Here's how the part is built. I have some questions about the finished solid (model axes, mm). A direction names the side the tool comes from. Round coordinates to 2 decimals unless told otherwise and drop trailing zeros. Loops run counter-clockwise (first coordinate to the right, second up) from the corner with the lowest first, then second, coordinate; pieces in that order, holes last. Notation, with made-up numbers: (6.25, 4.25) - (20.25, 4.25) arc R32 cw to (20.25, 40.25) - close; hole circle Ø2 at (49.5, 77). An arc over 180 degrees is marked (long way). Answer as a JSON object with one key per item and string values. Group by question number.
1) Will these pins go through, and if not, where does the flat tip stop? P1, Ø1.5, axis at y = 1.5, z = 1.5, coming from the -X side; P2, Ø0.9, axis at y = 2, z = 1.5, coming from the +X side; P3, Ø0.8, axis at x = 1.5, z = 1, coming from the -Y side.
2) I want a section at C-C, the plane y = 2.5. Please give me the cut outline in (x, z).
3) Which directions (+Z, -Z, +X, -X, +Y, -Y) give clear straight access to the entire face, cutting with the end or side of a thin tool? Please do faces 1 (the face through (1, 3, 1)), 2 (the face through (0, 14, 1)), 3 (the face through (7.75, 2, 1)).
4) If I drill on line 1 along X through (y, z) = (25, 0.7); line 2 along Y through (x, z) = (6.25, 2.3); line 3 along Y through (x, z) = (4.75, 2.05), over which ranges is the centre line in solid material (lowest first)? Write a range as [from, to].
5) I want a section at D-D, the plane x = 9.75. Please give me the cut outline in (y, z).
6) I want a section at A-A, the plane z = 1.6. Please give me the cut outline in (x, y), then the cut area to 3 significant figures.
7) If we mould it in two halves opening along X, with no side actions, what happens to faces 4 (the face through (9, 3, 1)), 5 (the face through (10.5, 14, 1)), 6 (the face through (5.3, 26.5, 1.5))? For each: pulls with the +X half, pulls with the -X half, needs draft (parallel to the pull), parting line crosses it, or undercut.
8) I want a section at B-B, the plane x = 4.75. Please give me the cut outline in (y, z), then the cut area to 3 significant figures.
from build123d import *

# Parameters (mm, degrees)
PLATE_THICKNESS_3MM_DEPTH = 3


with BuildPart() as part:
    # Sketch1 → Plate_thickness_3mm (new body)
    with BuildSketch(Plane.XY):
        with BuildLine():
            Line((10.5, 25), (10.5, 3))
            Line((10.5, 3), (7.75, 3))
            Line((7.75, 3), (7.75, 0))
            Line((7.75, 0), (2.75, 0))
            Line((2.75, 0), (2.75, 3))
            Line((2.75, 3), (0, 3))
            Line((0, 3), (0, 25))
            ThreePointArc((0, 25), (1.537689399, 28.712310601), (5.25, 30.25))
            ThreePointArc((5.25, 30.25), (8.962310601, 28.712310601), (10.5, 25))
        make_face()
        with BuildLine():
            ThreePointArc((5.25, 26.5), (3.75, 25), (5.25, 23.5))
            ThreePointArc((5.25, 23.5), (6.75, 25), (5.25, 26.5))
        make_face(mode=Mode.SUBTRACT)
    extrude(amount=PLATE_THICKNESS_3MM_DEPTH)


solid = part.part
Outcome:
{
 "1": {"P1": "x = 2.75", "P2": "x = 7.75", "P3": "y = 3"},
 "2": {"outline": "(2.75, 0) - (7.75, 0) - (7.75, 3) - (2.75, 3) - close"},
 "3": {"face 1": "+Z, -Z, -X, -Y", "face 2": "+Z, -Z, -X, +Y, -Y", "face 3": "+Z, -Z, +X, -Y"},
 "4": {"line 1": "[0, 3.75], [6.75, 10.5]", "line 2": "[0, 23.88], [26.12, 30.15]", "line 3": "[0, 23.59], [26.41, 30.23]"},
 "5": {"outline": "(3, 0) - (27.7, 0) - (27.7, 3) - (3, 3) - close"},
 "6": {"outline": "(0, 3) - (2.75, 3) - (2.75, 0) - (7.75, 0) - (7.75, 3) - (10.5, 3) - (10.5, 25) arc R5.25 ccw to (0, 25) - close; hole circle Ø3 at (5.25, 25)", "area": "282 mm^2"},
 "7": {"face 4": "needs draft", "face 5": "pulls with the +X half", "face 6": "undercut"},
 "8": {"outline": "(0, 0) - (23.59, 0) - (23.59, 3) - (0, 3) - close; (26.41, 0) - (30.23, 0) - (30.23, 3) - (26.41, 3) - close", "area": "82.2 mm^2"}
}
